Verification items for the finished model (mm, model axes). A direction names the side the tool comes from. Round coordinates to 2 decimals unless told otherwise and drop trailing zeros. Order: outer loops, then holes, each group sorted by start corner. A loop starts at its lowest first (then second) coordinate and runs counter-clockwise, first axis right, second up.
```python
from build123d import *

# Parameters (mm, degrees)
SKETCH1_W           = 20
SKETCH1_H           = 25.4
BOSS_EXTRUDE1_DEPTH = 10
SKETCH2_W           = 20
SKETCH2_H           = 10
BOSS_EXTRUDE2_DEPTH = 30
SKETCH3_R           = 3.81
CUT_EXTRUDE1_DEPTH  = 30
SKETCH4_R           = 2.54
CUT_EXTRUDE2_DEPTH  = 30


with BuildPart() as part:
    # Sketch1 → Boss-Extrude1 (new body)
    with BuildSketch(Plane(origin=(0, 0, 0), x_dir=(1, 0, 0), z_dir=(0, 1, 0))):
        with Locations((10, 12.7)):
            Rectangle(SKETCH1_W, SKETCH1_H)
    extrude(amount=BOSS_EXTRUDE1_DEPTH)

    # Sketch2 → Boss-Extrude2 (add)
    with BuildSketch(Plane(origin=(0, 0, 0), x_dir=(1, 0, 0), z_dir=(0, 1, 0))):
        with Locations((10, 30.4)):
            Rectangle(SKETCH2_W, SKETCH2_H)
    extrude(amount=BOSS_EXTRUDE2_DEPTH)

    # Sketch3 → Cut-Extrude1 (cut)
    with BuildSketch(Plane(origin=(0, 10, 0), x_dir=(1, 0, 0), z_dir=(0, 1, 0))):
        with Locations(Location((10, 6, 0), (0, 0, 270))):
            Circle(SKETCH3_R)
    extrude(amount=-CUT_EXTRUDE1_DEPTH, mode=Mode.SUBTRACT)

    # Sketch4 → Cut-Extrude2 (cut)
    with BuildSketch(Plane(origin=(0, 0, -35.4), x_dir=(-1, 0, 0), z_dir=(0, 0, -1))):
        with Locations((-10.522018302, 24)):
            Circle(SKETCH4_R)
        with Locations((-10.522018302, 15)):
            Circle(SKETCH4_R)
    extrude(amount=-CUT_EXTRUDE2_DEPTH, mode=Mode.SUBTRACT)


solid = part.part
```
1) Sectioned sample at A-A on z = -6. Record the cut outline in (x, y).
2) Go/stop test with flat-tipped pins: pin 1 Ø8 at (x, y) = (10.52, 15) entering from -Z; pin 2 Ø3 at (x, z) = (11.5, -14.5) entering from +Y; pin 3 Ø3 at (x, y) = (5, 20) entering from +Z. Record where each tip stops, or that it passes through.
3) Sectioned sample at C-C on x = 10.75. Record the cut outline in (y, z).
4) Sectioned sample at D-D on y = 8.75. Record the cut outline in (x, z).
5) Tool access check on faces 1 (the flat face through (10, 10, -13)), 2 (the flat face through (0, 8, -21)). Record the directions out of +Z, -Z, +X, -X, +Y, -Y that give a thin tool (end or side, any length) a straight path to the whole face; none if there is none.
6) Draft check along Y on faces 3 (the flat face through (7.6, 14.8, -35.4)), 4 (the flat face through (10, 0, -18)), 5 (the cylindrical face through (9.35, 12.747, -30.47)). Enter one of: released by +Y, released by -Y, zero draft, split by the parting line, or undercut.
7) Sectioned sample at B-B on y = 15. Record the cut outline in (x, z).
8) Scan lines: probe 1 along X at (y, z) = (2.5, -6); probe 2 along Z at (x, y) = (9.75, 18.75); probe 3 along Y at (x, z) = (11.75, -9.5). Record each from-to range of solid material in increasing order.
Returned:
1. outline: (0, 0) - (6.19, 0) - (6.19, 10) - (0, 10) - close; (13.81, 0) - (20, 0) - (20, 10) - (13.81, 10) - close
2. pin 1: stops at z = -35.4
2. pin 2: stops at y = 10
2. pin 3: stops at z = -25.4
3. outline: (0, -35.4) - (12.47, -35.4) - (12.47, -25.4) - (10, -25.4) - (10, -9.74) - (0, -9.74) - close; (0, -2.26) - (10, -2.26) - (10, 0) - (0, 0) - close; (17.53, -35.4) - (21.47, -35.4) - (21.47, -25.4) - (17.53, -25.4) - close; (26.53, -35.4) - (30, -35.4) - (30, -25.4) - (26.53, -25.4) - close
4. outline: (0, -35.4) - (20, -35.4) - (20, 0) - (0, 0) - close; hole circle Ø7.62 at (10, -6)
5. face 1: +Z, +X, -X, +Y
5. face 2: +Z, -Z, -X, +Y, -Y
6. face 3: zero draft
6. face 4: released by -Y
6. face 5: undercut
7. outline: (0, -35.4) - (7.98, -35.4) - (7.98, -25.4) - (0, -25.4) - close; (13.06, -35.4) - (20, -35.4) - (20, -25.4) - (13.06, -25.4) - close
8. probe 1: x = 0 to 6.19, 13.81 to 20
8. probe 2: z = -35.4 to -25.4
8. probe 3: y = 0 to 10
